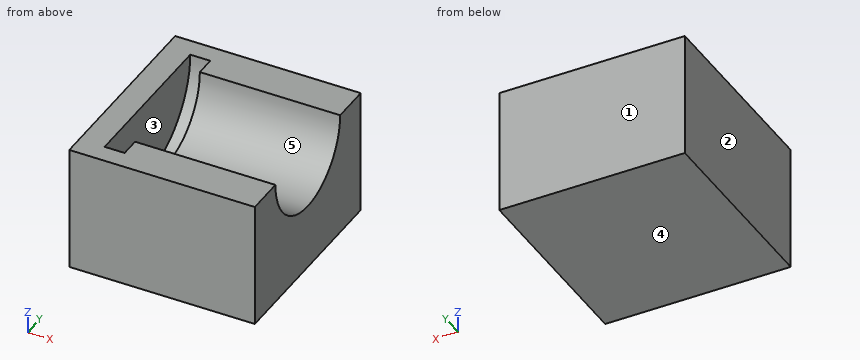
from build123d import *

# Parameters (mm, degrees)
F1_DEPTH  = 145
F2_W      = 15.7
F2_H      = 15
F3_DEPTH  = 11.463
F4_W      = 15.7
F4_H      = 15
F5_DEPTH  = 11.463
F7_DEPTH  = 25.427
F8_R      = 6.35
F8_R_2    = 4.8005
F9_DEPTH  = 1.5875
F10_R     = 6.35
F11_DEPTH = 1.5875
F12_W     = 129.3
F12_H     = 2.5
F12_H_2   = 15
F13_DEPTH = 25.427
F15_DEPTH = 25.427
F16_W     = 12.713
F16_H     = 10
F17_DEPTH = 15.701
F19_DEPTH = 2


with BuildPart() as f1:
    # F0 (on Front) → F1 (new body)
    with BuildSketch(Plane.XZ):
        Polygon((0, 2.5), (0, 0), (12.713, 0), (25.426, 0), (25.426, 2.5), (13.963, 2.5), (13.963, 17.5), (25.426, 17.5), (25.426, 20), (12.713, 20), (0, 20), (0, 17.5), (11.463, 17.5), (11.463, 2.5), align=None)
    extrude(amount=-F1_DEPTH)

    # F2 (on face) → F3 (join, through all)
    with BuildSketch(Plane.YZ.offset(13.963)):
        with Locations((7.85, 10)):
            Rectangle(F2_W, F2_H)
    extrude(amount=F3_DEPTH)

    # F4 (on face) → F5 (join, through all)
    with BuildSketch(Plane(origin=(11.463, 0, 0), x_dir=(0, -1, 0), z_dir=(-1, 0, 0))):
        with Locations((-7.85, 10)):
            Rectangle(F4_W, F4_H)
    extrude(amount=F5_DEPTH)

    # F6 (on face) → F7 (cut, through all)
    with BuildSketch(Plane.YZ.offset(25.426)):
        with BuildLine():
            Line((3.0495, 10), (12.6505, 10))
            ThreePointArc((12.6505, 10), (7.85, 14.8005), (3.0495, 10))
        make_face()
        with BuildLine():
            ThreePointArc((3.0495, 10), (7.85, 5.1995), (12.6505, 10))
            Line((12.6505, 10), (3.0495, 10))
        make_face()
    extrude(amount=-F7_DEPTH, mode=Mode.SUBTRACT)

    # F8 (on face) → F9 (cut)
    with BuildSketch(Plane.YZ.offset(25.426)):
        with Locations((7.85, 10)):
            Circle(F8_R)
        with Locations((7.85, 10)):
            Circle(F8_R_2, mode=Mode.SUBTRACT)
    extrude(amount=-F9_DEPTH, mode=Mode.SUBTRACT)

    # F10 (on face) → F11 (cut)
    with BuildSketch(Plane(origin=(0, 0, 0), x_dir=(0, -1, 0), z_dir=(-1, 0, 0))):
        with Locations((-7.85, 10)):
            Circle(F10_R)
    extrude(amount=-F11_DEPTH, mode=Mode.SUBTRACT)

    # F12 (on face) → F13 (cut, through all)
    with BuildSketch(Plane.YZ.offset(25.426)):
        with Locations((80.35, 18.75)):
            Rectangle(F12_W, F12_H)
        with Locations((80.35, 10)):
            Rectangle(F12_W, F12_H_2)
        with Locations((80.35, 1.25)):
            Rectangle(F12_W, F12_H)
    extrude(amount=-F13_DEPTH, mode=Mode.SUBTRACT)

    # F14 (on face) → F15 (cut, through all)
    with BuildSketch(Plane(origin=(0, 0, 0), x_dir=(0, -1, 0), z_dir=(-1, 0, 0))):
        with BuildLine():
            ThreePointArc((-14.2, 10), (-7.85, 16.35), (-1.5, 10))
            Line((-1.5, 10), (0, 10))
            Line((0, 10), (0, 20))
            Line((0, 20), (-15.7, 20))
            Line((-15.7, 20), (-15.7, 10))
            Line((-15.7, 10), (-14.2, 10))
        make_face()
        with BuildLine():
            Line((-14.2, 10), (-1.5, 10))
            ThreePointArc((-1.5, 10), (-7.85, 16.35), (-14.2, 10))
        make_face()
    extrude(amount=-F15_DEPTH, mode=Mode.SUBTRACT)

    # F16 (on face) → F17 (cut, through all)
    with BuildSketch(Plane.XZ):
        with Locations((19.0695, 5)):
            Rectangle(F16_W, F16_H)
    extrude(amount=-F17_DEPTH, mode=Mode.SUBTRACT)

    # F18 (on face) → F19 (join)
    with BuildSketch(Plane(origin=(0, 0, 0), x_dir=(0, -1, 0), z_dir=(-1, 0, 0))):
        with BuildLine():
            Line((-14.2, 10), (-15.7, 10))
            Line((-15.7, 10), (-15.7, 0))
            Line((-15.7, 0), (0, 0))
            Line((0, 0), (0, 10))
            Line((0, 10), (-1.5, 10))
            ThreePointArc((-1.5, 10), (-7.85, 3.65), (-14.2, 10))
        make_face()
        with BuildLine():
            Line((-1.5, 10), (-14.2, 10))
            ThreePointArc((-14.2, 10), (-7.85, 3.65), (-1.5, 10))
        make_face()
    extrude(amount=F19_DEPTH)


solid = f1.part
Here's how the part is built. I have some questions about the finished solid (model axes, mm). Face numbers are marked on the shaded views. A direction names the side the tool comes from. Coordinates: 2 decimals unless noted, no trailing zeros. Order: outer loops, then holes, each group sorted by start corner. A loop starts at its lowest first (then second) coordinate and runs counter-clockwise, first axis right, second up. Notation, with made-up numbers: M 41,-17.5 L 48,-17.5 A23 cw 48,10.5 Z; hole C -3,51.5 d7. An arc over 180 degrees is marked long. Answer as CSV lines item,"result". Start each with the question number.
1. We'd pull the mould along Y, two halves only. Please class the marked faces 1, 2 and 3: released by +Y, released by -Y, zero draft, split by the parting line, or undercut.
2. I want a section at C-C, the plane z = 8.25. Write out the boundary of the cut face in (x, y).
3. On a 3-axis mill with a long thin cutter (end or side, diameter ignored), from which of +Z, -Z, +X, -X, +Y, -Y can I reach the whole of each face in a straight line? I mean the marked faces 4 and 5. Say none if no direction works.
4. I need wall thicknesses on line 1 (X direction, y = 13.5, z = 7.75); line 2 (Y direction, x = 1.5, z = 7); line 3 (Z direction, x = 5.5, y = 7.75). Which ranges of each line are inside material? Lowest first, please. Write a range as [from, to].
5. I want a section at D-D, the plane y = 13.5. Write out the boundary of the cut face in (x, z), and give its area (3 significant figures).
6. I want a section at B-B, the plane x = 6. Write out the boundary of the cut face in (y, z), and give its area (3 significant figures).
7. I want a section at A-A, the plane y = 7.85. Write out the boundary of the cut face in (x, z).
8. For pin 1 (3 mm diameter, centred on y = 5.5, z = 8, fed in from +X), with a flat end and sliding along its axis, tell me the tip position at first contact or that it passes through.
Recorded:
1,face 1,"released by +Y"
1,face 2,"zero draft"
1,face 3,"undercut"
2,outline,"M -2,0 L 12.71,0 L 12.71,3.38 L 1.59,3.38 L 1.59,1.75 L 0,1.75 L 0,13.95 L 1.59,13.95 L 1.59,12.32 L 12.71,12.32 L 12.71,15.7 L -2,15.7 Z"
3,face 4,"-Z, +X, -X, +Y, -Y"
3,face 5,"+Z, +X"
4,line 1,"x = [-2, 0], [1.59, 12.71]"
4,line 2,"y = [0, 2.25], [13.45, 15.7]"
4,line 3,"z = [0, 5.2]"
5,outline,"M -2,0 L 12.71,0 L 12.71,10 L 1.59,10 L 1.59,7.1 L 0,7.1 L 0,10 L -2,10 Z"
5,area,"143 mm2"
6,outline,"M 0,0 L 15.7,0 L 15.7,10 L 12.65,10 A4.8 cw 3.05,10 L 0,10 Z"
6,area,"121 mm2"
7,outline,"M -2,0 L 12.71,0 L 12.71,5.2 L 1.59,5.2 L 1.59,3.65 L 0,3.65 L 0,10 L -2,10 Z"
8,pin 1,"stops at x = 0"
